Geometry check sheet. Reference: the model listing, model coordinates, mm. Face numbers are marked on the shaded views. A direction names the side the tool comes from. Coordinates: 2 decimals unless noted, no trailing zeros. Write each loop counter-clockwise with the first axis right and the second up, starting at its lowest first coordinate (ties: lowest second). Pieces come first, ordered by that corner, then holes. Notation, with made-up numbers: M 57,57.5 L 115,57.5 A24 ccw 115,68.5 Z; hole C 14.5,22 d6. An arc over 180 degrees is marked long. Answer as a JSON object with one key per item and string values. Group by question number.
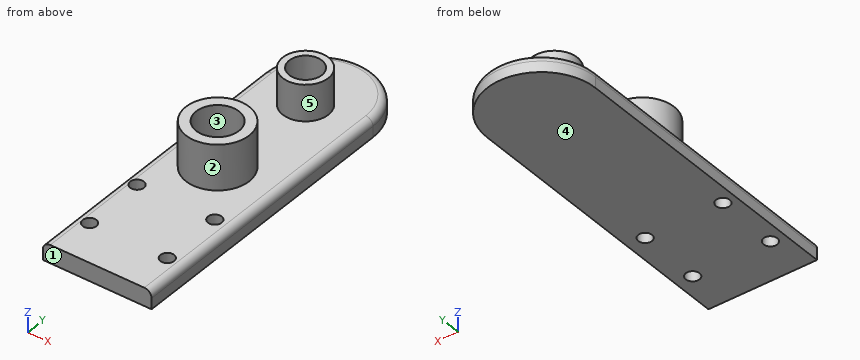
```python
from build123d import *

# Parameters (mm, degrees)
F1_DEPTH     = 12.7
F2_R         = 4.826
F3_DEPTH     = 12.701
F4_R         = 22.225
F5_DEPTH     = 31.75
F6_R         = 16.002
F6_R_2       = 11.4285628251
F7_DEPTH     = 25.4
F8_R         = 15.0651318588
F9_DEPTH     = 31.75
F10_T1_DEPTH = 215.9
F10_T4_ANGLE = 180


# Not quite as in the source:
# - a fillet or chamfer that OpenCascade refuses, or shapes differently, is made with other operations: its cross-section is extruded or revolved along the edge and cut away or added


with BuildPart() as f1:
    # F0 (on Top) → F1 (new body)
    with BuildSketch(Plane.XY):
        with BuildLine():
            Line((-28.8097388059, 45.6853893078), (-28.8097388059, -157.5146106922))
            Line((-28.8097388059, -157.5146106922), (47.3902611941, -157.5146106922))
            Line((47.3902611941, -157.5146106922), (47.3902611941, 45.6853893078))
            ThreePointArc((47.3902611941, 45.6853893078), (9.2902611941, 83.7853893078), (-28.8097388059, 45.6853893078))
        make_face()
    extrude(amount=F1_DEPTH)

    # F2 (on face) → F3 (cut, through all)
    with BuildSketch(Plane.XY.offset(12.7)):
        with Locations((-18.8133654982, -127.8345082872)):
            Circle(F2_R)
        with Locations((35.5419658125, -127.5648898334)):
            Circle(F2_R)
        with Locations((-19.6402604571, -83.1381565264)):
            Circle(F2_R)
        with Locations((34.7150708535, -82.8685380725)):
            Circle(F2_R)
    extrude(amount=-F3_DEPTH, mode=Mode.SUBTRACT)

    # F4 (on face) → F5 (join)
    with BuildSketch(Plane.XY.offset(12.7)):
        with Locations((5.8846990578, -42.6385067403)):
            Circle(F4_R)
    extrude(amount=F5_DEPTH)

    # F6 (on face) → F7 (join)
    with BuildSketch(Plane.XY.offset(12.7)):
        with Locations((9.203276597, 33.7460897863)):
            Circle(F6_R)
        with Locations((9.203276597, 33.7460897863)):
            Circle(F6_R_2, mode=Mode.SUBTRACT)
    extrude(amount=F7_DEPTH)

    # F8 (on face) → F9 (cut)
    with BuildSketch(Plane.XY.offset(44.45)):
        with Locations((5.8846990578, -42.6385067403)):
            Circle(F8_R)
    extrude(amount=-F9_DEPTH, mode=Mode.SUBTRACT)

    # F10: fillet of radius 5.08 on 3 edges, made by hand

    # F10_s2 → F10_t1 (cut)
    with BuildSketch(Plane.XZ.offset(-45.6853893078)):
        with BuildLine():
            ThreePointArc((42.3102611941, 12.7), (45.9023636425, 11.2121024484), (47.3902611941, 7.62))
            Line((47.3902611941, 7.62), (47.3902611941, 12.7))
            Line((47.3902611941, 12.7), (42.3102611941, 12.7))
        make_face()
        with BuildLine():
            ThreePointArc((-28.8097388059, 7.62), (-27.3218412543, 11.2121024484), (-23.7297388059, 12.7))
            Line((-23.7297388059, 12.7), (-28.8097388059, 12.7))
            Line((-28.8097388059, 12.7), (-28.8097388059, 7.62))
        make_face()
    extrude(amount=F10_T1_DEPTH, mode=Mode.SUBTRACT)

    # F10_s3 → F10_t4 (revolve, cut)
    with BuildSketch(Plane.XZ.offset(-45.6853893078)):
        with BuildLine():
            ThreePointArc((47.3902611941, 7.62), (45.9023636425, 11.2121024484), (42.3102611941, 12.7))
            Line((42.3102611941, 12.7), (47.3902611941, 12.7))
            Line((47.3902611941, 12.7), (47.3902611941, 7.62))
        make_face()
    revolve(axis=Axis((9.2902611941, 45.6853893078, 12.7), (0, 0, 1)), revolution_arc=F10_T4_ANGLE, mode=Mode.SUBTRACT)


solid = f1.part
```
1) Material ranges on probe 1 along Y at (x, z) = (-18, 2); probe 2 along Z at (x, y) = (16, -53.5); probe 3 along Y at (x, z) = (16.5, 14.5), recorded low to high. Write a range as [from, to].
2) Section check C-C (z = 23.5). State how many separate pieces and enclosed holes the cut face has, then the cut area to 3 significant figures.
3) Go/stop test with flat-tipped pins: pin 1 Ø20 at (x, y) = (9, -93) entering from +Z; pin 2 Ø10 at (x, z) = (-6.5, 16.5) entering from +Y (3 decimals); pin 3 Ø1.5 at (x, z) = (20, 32) entering from +Y. Record where each tip stops, or that it passes through.
4) Section check B-B (z = 3). Record the cut outline in (x, y).
5) Section check A-A (y = -130). Record the cut outline in (x, z), then the cut area to 3 significant figures.
6) Draft check along X on the marked faces 3, 4 and 5. Enter one of: +X half, -X half, draft (parallel to the pull), parting line (faces both ways), or undercut.
7) Set-up check for the marked faces 1 and 2: record each of +Z, -Z, +X, -X, +Y, -Y from which the full face is reachable in a straight line by a thin tool's end or side.
8) Section check D-D (y = -25.5). Record the cut outline in (x, z), then the cut area to 3 significant figures.
Entries:
{
 "1": {"probe 1": "[-157.51, -132.59], [-123.08, -87.68], [-78.6, 72.27]", "probe 2": "[0, 12.7]", "probe 3": "[-62.16, -53.33], [-31.95, -23.11], [19.5, 24.95], [42.54, 47.99]"},
 "2": {"separate pieces": "2", "enclosed holes": "2", "area": "1,230 mm^2"},
 "3": {"pin 1": "z = 12.7", "pin 2": "y = 78.735", "pin 3": "y = 46.2"},
 "4": {"outline": "M -28.81,-157.51 L 47.39,-157.51 L 47.39,45.69 A38.1 ccw -28.81,45.69 Z; hole C -19.64,-83.14 d9.65; hole C -18.81,-127.83 d9.65; hole C 34.72,-82.87 d9.65; hole C 35.54,-127.56 d9.65"},
 "5": {"outline": "M -28.81,0 L -23.13,0 L -23.13,12.7 L -23.73,12.7 A5.08 ccw -28.81,7.62 Z; M -14.5,0 L 31.38,0 L 31.38,12.7 L -14.5,12.7 Z; M 39.71,0 L 47.39,0 L 47.39,7.62 A5.08 ccw 42.31,12.7 L 39.71,12.7 Z", "area": "741 mm^2"},
 "6": {"face 3": "undercut", "face 4": "draft", "face 5": "parting line"},
 "7": {"face 1": "+Z, -Z, +X, -X, -Y", "face 2": "+Z"},
 "8": {"outline": "M -28.81,0 L 47.39,0 L 47.39,7.62 A5.08 ccw 42.31,12.7 L 20.03,12.7 L 20.03,44.45 L -8.27,44.45 L -8.27,12.7 L -23.73,12.7 A5.08 ccw -28.81,7.62 Z", "area": "1,860 mm^2"}
}
